Read the model definition and answer for the solid it produces. Units are mm, in the model's axes. Face numbers are marked on the shaded views. A direction names the side the tool comes from. Give positions to 0.01 mm unless a question says otherwise; leave off trailing zeros. Loops run counter-clockwise (first coordinate to the right, second up) from the corner with the lowest first, then second, coordinate; pieces in that order, holes last. Notation, with made-up numbers: (43, 20) - (87, 20) arc R23 ccw to (87, 43) - close; hole circle Ø10 at (-12, -32). An arc over 180 degrees is marked (long way). Write item = value, one per line. Start each with the question number.
from build123d import *

# Parameters (mm, degrees)
F1_DEPTH = 500
F2_R     = 5.25
F3_DEPTH = 10
F4_R     = 5.25
F5_DEPTH = 10


with BuildPart() as f1:
    # F0 (on Top) → F1 (new body)
    with BuildSketch(Plane.XY):
        Polygon((-25, 30), (-30, 30), (-30, -30), (30, -30), (30, -25), (-25, -25), align=None)
    extrude(amount=-F1_DEPTH)

    # F2 (on face) → F3 (cut)
    with BuildSketch(Plane.XZ.offset(30)):
        with Locations((0, -20)):
            Circle(F2_R)
        with Locations((0, -100)):
            Circle(F2_R)
    extrude(amount=-F3_DEPTH, mode=Mode.SUBTRACT)

    # F4 (on face) → F5 (cut)
    with BuildSketch(Plane(origin=(-30, 0, 0), x_dir=(0, -1, 0), z_dir=(-1, 0, 0))):
        with Locations((0, -20)):
            Circle(F4_R)
        with Locations((0, -100)):
            Circle(F4_R)
    extrude(amount=-F5_DEPTH, mode=Mode.SUBTRACT)


solid = f1.part
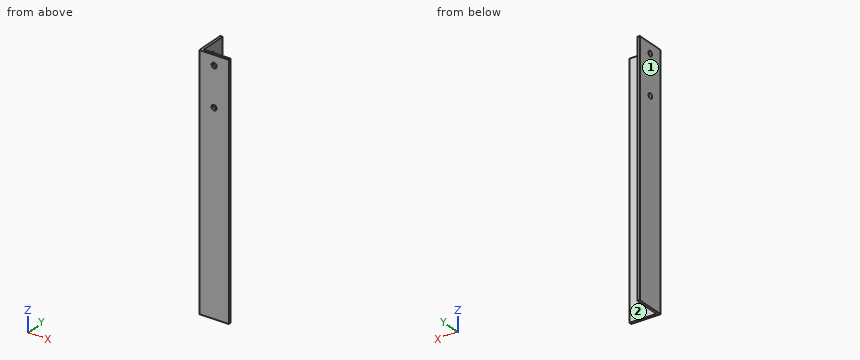
1. A cutting plane is placed at C-C on z = -20. Give the vertices of the cut face in (x, y).
2. Given P1, Ø5, axis at x = -10.5, z = -298.5, coming from the +Y side; P2, Ø5, axis at y = -20.5, z = -308.5, coming from the +X side; P3, Ø8.5, axis at x = 0, z = -100, coming from the -Y side, each flat-ended and moving along its own axis, determine where each tip first touches the part or whether it passes through.
3. A tool of negligible diameter and unlimited length cuts with its end or side. For the marked faces 1 and 2, from which of +Z, -Z, +X, -X, +Y, -Y can it reach the whole face along a straight path? Write none if from no direction.
4. A cutting plane is placed at D-D on z = -301. Give the vertices of the cut face in (x, y).
5. Consider line 1 along Z through (x, y) = (-27, 0); line 2 along X through (y, z) = (26, -122). Determine where each line is inside the solid, lowest interval first. Write a range as [from, to].
6. A cutting plane is placed at A-A on x = 0. Give the vertices of the cut face in (y, z), and give its area (4 significant figures).
Reply:
q1.outline = (-30, -30) - (-5.25, -30) - (-5.25, -25) - (-25, -25) - (-25, -5.25) - (-30, -5.25) - close; (-30, 5.25) - (-25, 5.25) - (-25, 30) - (-30, 30) - close; (5.25, -30) - (30, -30) - (30, -25) - (5.25, -25) - close
q2.P1 = -25
q2.P2 = -25
q2.P3 = through
q3.face_1 = +Z, -Z, -X, +Y, -Y
q3.face_2 = +Z, -Z, +X, +Y
q4.outline = (-30, -30) - (30, -30) - (30, -25) - (-25, -25) - (-25, 30) - (-30, 30) - close
q5.line_1 = [-500, -105.25], [-94.75, -25.25], [-14.75, 0]
q5.line_2 = [-30, -25]
q6.outline = (-30, -500) - (-25, -500) - (-25, -105.25) - (-30, -105.25) - close; (-30, -94.75) - (-25, -94.75) - (-25, -25.25) - (-30, -25.25) - close; (-30, -14.75) - (-25, -14.75) - (-25, 0) - (-30, 0) - close
q6.area = 2,395 mm^2
